Autodesk Inventor part; units mm, degrees
ref_plane "YZ Plane" through (0, 0, 0) normal (1, 0, 0) x (0, 1, 0)
ref_plane "XZ Plane" through (0, 0, 0) normal (0, 1, 0) x (-1, 0, 0)
ref_plane "XY Plane" through (0, 0, 0) normal (0, 0, 1) x (1, 0, 0)
sketch "Sketch1" plane through (0, 0, 0) normal (0, 0, 1) x (1, 0, 0)
  circle A0 centre (0, 0) radius 6.35
  circle A1 centre (0, 0) radius 7.9375
  circle A2 centre (0, 0) radius 9.525
  dimension "d0" = 12.7
  dimension "d1" = 15.875
  dimension "d2" = 19.05
extrude "Extrusion1" add sketch "Sketch1" against normal blind 9.525 contours A1
extrude "Extrusion2" add sketch "Sketch1" along normal blind 1.5875 contours A1 | A2
chamfer "Chamfer1" distance 0.254 angle 45 3 edges at (-9.525, 0, 1.5875) (-6.35, 0, 1.5875) (-6.35, 0, -9.525)
properties part number "Chassis_Washer_AndyMark_am-0947" material "Nylon-6/6"
Geometry: final body of the model. Coordinates: model frame, mm. A direction names the side the tool comes from. Coordinates: 2 decimals unless noted, no trailing zeros. Put each result on its own line as item: value.
(1) Material intervals for probe 1 along Y at (x, z) = (0, -5.25); probe 2 along Y at (x, z) = (2.25, -0.75); probe 3 along Z at (x, y) = (0.5, 8.75), sorted ascending.
Answer sheet:
probe 1: y = -7.94 to -6.35, 6.35 to 7.94
probe 2: y = -7.61 to -5.94, 5.94 to 7.61
probe 3: z = 0 to 1.59
(2) First-contact query: pin 1 (2 mm diameter, centred on x = -1.5, z = -5.5, fed in from -Y); pin 2 (4 mm diameter, centred on x = -3, z = -0.5, fed in from +Y); pin 3 (3 mm diameter, centred on x = 4.5, z = -4, fed in from +Y); pin 4 (10 mm diameter, centred on x = 0, y = 0, fed in from -Z) (3 decimals). Flat tips, straight axial feed; report the tip coordinate or a pass-through.
Answer sheet:
pin 1: stops at y = -7.92
pin 2: stops at y = 9.47
pin 3: stops at y = 7.35
pin 4: passes through
(3) Draft query along Y for faces 1 (the face through (-1.38, -6.2, -3.89)), 2 (the face through (-7.559, 5.796, 0.657)), 3 (the face through (-2, 7, -9.525)). Return one class per face: pulls with the +Y half, pulls with the -Y half, needs draft (parallel to the pull), parting line crosses it, or undercut.
Answer sheet:
face 1: undercut
face 2: parting line crosses it
face 3: needs draft
(4) Access query for faces 4 (the face through (-2, 8, 0)), 5 (the face through (4, -6, 1.588)). Directions: +Z, -Z, +X, -X, +Y, -Y. A direction counts if a zero-diameter tool reaches every point of the face in a straight line with its end or side. Return the directions, or none.
Answer sheet:
face 4: -Z
face 5: +Z, +X, -X, +Y, -Y
